Input: part model. Units: mm. Frame: model coordinates. A direction names the side the tool comes from. Round coordinates to 2 decimals unless told otherwise and drop trailing zeros. Loops run counter-clockwise (first coordinate to the right, second up) from the corner with the lowest first, then second, coordinate; pieces in that order, holes last.
1) Access query for faces 4 (the face through (9.43, 37.4, 0.5)), 5 (the face through (-13.9, -59.43, 0.5)). Directions: +Z, -Z, +X, -X, +Y, -Y. A direction counts if a zero-diameter tool reaches every point of the face in a straight line with its end or side. Return the directions, or none.
2) Section A-A, the plane y = 26. Return loops of the section in (x, z).
3) Draft query along Y for faces 1 (the face through (-13.93, 59.4, 0.5)), 2 (the face through (8.583, -52.795, 0.501)), 3 (the face through (-6, 1, 0)). Return one class per face: pulls with the +Y half, pulls with the -Y half, needs draft (parallel to the pull), parting line crosses it, or undercut.
4) Section B-B, the plane y = 42.5. Return loops of the section in (x, z).
5) Section C-C, the plane z = 0.3. State how many separate pieces and enclosed holes the cut face has, and give its area (3 significant figures).
6) Ray query, line 1 along X through (y, z) = (-43.5, 0.5); line 2 along X through (y, z) = (5, 0.7); line 3 along X through (y, z) = (49.5, 0.5). Return the intervals inside material, ascending.
from build123d import *

# Parameters (mm, degrees)
BOSS_EXTRUDE4_DEPTH    = 1.016
CUT_EXTRUDE2_OUTLINE_W = 3.7
CUT_EXTRUDE2_OUTLINE_H = 1
CUT_EXTRUDE2_DEPTH     = 1.016


with BuildPart() as part:
    # Sketch6 → Boss-Extrude4 (new body)
    with BuildSketch(Plane.XY):
        with BuildLine():
            Line((-12.5, 60), (4.5, 60))
            ThreePointArc((4.5, 60), (11.571067812, 57.071067812), (14.5, 50))
            Line((14.5, 50), (14.5, -58))
            ThreePointArc((14.5, -58), (13.914213562, -59.414213562), (12.5, -60))
            Line((12.5, -60), (-12.5, -60))
            ThreePointArc((-12.5, -60), (-13.914213562, -59.414213562), (-14.5, -58))
            Line((-14.5, -58), (-14.5, 58))
            ThreePointArc((-14.5, 58), (-13.914213562, 59.414213562), (-12.5, 60))
        make_face()
    extrude(amount=BOSS_EXTRUDE4_DEPTH)

    # Cut-Extrude2: read off the stored shape, not the designer's step
    # Cut-Extrude2 outline → Cut-Extrude2 (cut)
    with BuildSketch(Plane.XY):
        with BuildLine():
            add(Edge.make_bspline(
                [(0.464136716, -29.280008599), (0.50069296, -29.588797386), (0.532256612, -29.958993284), (0.568812856, -30.267782071)],
                knots=[2, 2, 2, 2, 3, 3, 3, 3], degree=3))
            add(Edge.make_bspline(
                [(0.464136716, -29.280008599), (0.460815442, -29.004347325), (0.24608723, -28.738291079), (4.711e-06, -28.733078818)],
                knots=[25.000001953, 25.000001953, 25.000001953, 25.000001953, 25.984659899, 25.984659899, 25.984659899, 25.984659899], degree=3))
            add(Edge.make_bspline(
                [(-0.464136716, -29.280008613), (-0.460815442, -29.004347325), (-0.24608723, -28.738291079), (4.711e-06, -28.733078818)],
                knots=[25.000001953, 25.000001953, 25.000001953, 25.000001953, 25.984659899, 25.984659899, 25.984659899, 25.984659899], degree=3))
            Line((-0.464136716, -29.280008613), (-0.568812856, -30.267782071))
            Line((-0.568812856, -30.267782071), (-4.892180174, -41.831826427))
            Line((-4.892180174, -41.831826427), (-5.117963119, -42.406855927))
            Line((-5.117963119, -42.406855927), (-5.25555162, -43.003051232))
            Line((-5.25555162, -43.003051232), (-5.354849178, -43.616881121))
            Line((-5.354849178, -43.616881121), (-5.355849178, -44.579979095))
            Line((-5.355849178, -44.579979095), (-4.925, -48.85))
            Line((-4.925, -48.85), (-2.6, -49.6))
            Line((-2.6, -49.6), (-0.625, -49.6))
            Line((-0.625, -49.6), (-0.625, -51.23))
            Line((-0.625, -51.23), (0.625, -51.23))
            Line((0.625, -51.23), (0.625, -49.6))
            Line((0.625, -49.6), (2.6, -49.6))
            Line((2.6, -49.6), (4.925, -48.85))
            Line((4.925, -48.85), (5.332817408, -44.579979095))
            Line((5.332817408, -44.579979095), (5.328817408, -43.616881121))
            Line((5.328817408, -43.616881121), (5.232524742, -43.003051232))
            Line((5.232524742, -43.003051232), (5.094957773, -42.406855927))
            Line((5.094957773, -42.406855927), (4.862112382, -41.831826427))
            Line((4.862112382, -41.831826427), (0.568812856, -30.267782071))
        make_face()
        with BuildLine():
            ThreePointArc((4, 16.031829774), (3.443502884, 17.375332658), (2.1, 17.931829774))
            Line((2.1, 17.931829774), (-2.1, 17.931829774))
            ThreePointArc((-2.1, 17.931829774), (-3.443502884, 17.375332658), (-4, 16.031829774))
            Line((-4, 16.031829774), (-4, 1.6))
            ThreePointArc((-4, 1.6), (-3.443502884, 0.256497116), (-2.1, -0.3))
            Line((-2.1, -0.3), (2.1, -0.3))
            ThreePointArc((2.1, -0.3), (3.443502884, 0.256497116), (4, 1.6))
            ThreePointArc((4, 1.6), (4.602950898, 2.981782106), (5.999374902, 3.55))
            Line((5.999374902, 3.55), (7.000625098, 3.55))
            ThreePointArc((7.000625098, 3.55), (8.432407204, 2.946424004), (9, 1.5))
            Line((9, 1.5), (9, -0.435932815))
            Line((9, -0.435932815), (10.73, -5.355496174))
            Line((10.73, -5.355496174), (10.73, -7.27))
            Line((10.73, -7.27), (7.140268475, -7.27))
            Line((7.140268475, -7.27), (7.140268475, -9.27))
            Line((7.140268475, -9.27), (10.73, -9.27))
            Line((10.73, -9.27), (10.73, -48.528487843))
            ThreePointArc((10.73, -48.528487843), (10.644281066, -48.921574831), (10.402688829, -49.243286359))
            Line((10.402688829, -49.243286359), (6.339155629, -52.75))
            Line((6.339155629, -52.75), (-0.390660403, -52.75))
            ThreePointArc((-0.390660403, -52.75), (-0.96294992, -52.98705008), (-1.2, -53.559339597))
            Line((-1.2, -53.559339597), (-1.2, -53.640660403))
            ThreePointArc((-1.2, -53.640660403), (-0.96294992, -54.21294992), (-0.390660403, -54.45))
            Line((-0.390660403, -54.45), (6.665142853, -54.45))
            Line((6.665142853, -54.45), (10.556020375, -51.092283301))
            ThreePointArc((10.556020375, -51.092283301), (11.422548586, -49.938388133), (11.73, -48.528487843))
            Line((11.73, -48.528487843), (11.73, -5.184791238))
            Line((11.73, -5.184791238), (10, -0.265227879))
            Line((10, -0.265227879), (10, 36))
            ThreePointArc((10, 36), (9.414213562, 37.414213562), (8, 38))
            Line((8, 38), (6, 38))
            ThreePointArc((6, 38), (4.585786438, 38.585786438), (4, 40))
            Line((4, 40), (4, 54.1))
            ThreePointArc((4, 54.1), (3.443502884, 55.443502884), (2.1, 56))
            Line((2.1, 56), (-2.1, 56))
            ThreePointArc((-2.1, 56), (-3.443502884, 55.443502884), (-4, 54.1))
            Line((-4, 54.1), (-4, 38.9))
            ThreePointArc((-4, 38.9), (-3.443502884, 37.556497116), (-2.1, 37))
            Line((-2.1, 37), (8, 37))
            ThreePointArc((8, 37), (8.707106781, 36.707106781), (9, 36))
            Line((9, 36), (9, 6.55))
            ThreePointArc((9, 6.55), (8.414213562, 5.135786438), (7, 4.55))
            Line((7, 4.55), (6, 4.55))
            ThreePointArc((6, 4.55), (4.585786438, 5.135786438), (4, 6.55))
            Line((4, 6.55), (4, 16.031829774))
        make_face()
        with Locations((3.375465258, -8.27)):
            Rectangle(CUT_EXTRUDE2_OUTLINE_W, CUT_EXTRUDE2_OUTLINE_H)
    extrude(amount=CUT_EXTRUDE2_DEPTH, mode=Mode.SUBTRACT)


solid = part.part
Final values:
1. face 4: +Z, -Z
1. face 5: +Z, -Z, -X, -Y
2. outline: (-14.5, 0) - (9, 0) - (9, 1.02) - (-14.5, 1.02) - close; (10, 0) - (14.5, 0) - (14.5, 1.02) - (10, 1.02) - close
3. face 1: pulls with the +Y half
3. face 2: undercut
3. face 3: needs draft
4. outline: (-14.5, 0) - (-4, 0) - (-4, 1.02) - (-14.5, 1.02) - close; (4, 0) - (14.5, 0) - (14.5, 1.02) - (4, 1.02) - close
5. separate pieces: 1
5. enclosed holes: 3
5. area: 2,880 mm2
6. line 1: x = -14.5 to -5.34, 5.31 to 10.73, 11.73 to 14.5
6. line 2: x = -14.5 to -4, 4.74 to 8.26, 10 to 14.5
6. line 3: x = -14.5 to -4, 4 to 14.5
